Check sheet for the modelled part. Datum: model origin and axes. Units: mm. Give positions to 0.01 mm unless a question says otherwise; leave off trailing zeros. Loops run counter-clockwise (first coordinate to the right, second up) from the corner with the lowest first, then second, coordinate; pieces in that order, holes last. Notation, with made-up numbers: M 44,89.5 L 95,89.5 A6 ccw 95,95.5 Z; hole C -25.5,-27.75 d9. An arc over 180 degrees is marked long. Use one line per item in the form item = value.
from build123d import *

# Parameters (mm, degrees)
SKETCH1_R           = 67.5
SKETCH1_R_2         = 2.5
BOSS_EXTRUDE1_DEPTH = 7
SKETCH3_R           = 3
CUT_EXTRUDE1_DEPTH  = 10


with BuildPart() as part:
    # Sketch1 → Boss-Extrude1 (new body)
    with BuildSketch(Plane(origin=(0, 0, 0), x_dir=(1, 0, 0), z_dir=(0, 1, 0))):
        with Locations(Location((0, 0, 0), (0, 0, 270))):
            Circle(SKETCH1_R)
        with Locations(Location((-40, 23.094010768, 0), (0, 0, 270))):
            Circle(SKETCH1_R_2, mode=Mode.SUBTRACT)
        with Locations(Location((40, 23.094010768, 0), (0, 0, 270))):
            Circle(SKETCH1_R_2, mode=Mode.SUBTRACT)
        with Locations(Location((0, -46.188021535, 0), (0, 0, 270))):
            Circle(SKETCH1_R_2, mode=Mode.SUBTRACT)
    extrude(amount=BOSS_EXTRUDE1_DEPTH)

    # Sketch3 → Cut-Extrude1 (cut)
    with BuildSketch(Plane(origin=(0, 7, 0), x_dir=(1, 0, 0), z_dir=(0, 1, 0))):
        with Locations(Location((42.425, 42.425, 0), (0, 0, 270))):
            Circle(SKETCH3_R)
        with Locations(Location((42.425, -42.425, 0), (0, 0, 270))):
            Circle(SKETCH3_R)
        with Locations(Location((-42.425, -42.425, 0), (0, 0, 270))):
            Circle(SKETCH3_R)
        with Locations(Location((-42.425, 42.425, 0), (0, 0, 270))):
            Circle(SKETCH3_R)
    extrude(amount=-CUT_EXTRUDE1_DEPTH, mode=Mode.SUBTRACT)


solid = part.part
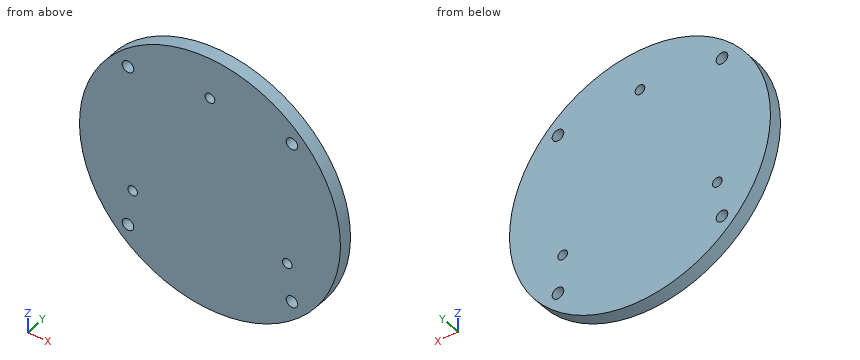
1) Section check A-A (y = 5.5). Record the cut outline in (x, z) (3 decimals), then the cut area to 3 significant figures.
Evaluation:
outline = C 0,0 d135; hole C -42.425,-42.425 d6; hole C -42.425,42.425 d6; hole C -40,-23.094 d5; hole C 0,46.188 d5; hole C 40,-23.094 d5; hole C 42.425,-42.425 d6; hole C 42.425,42.425 d6
area = 14,100 mm^2
2) Section check B-B (x = 54). Record the cut outline in (y, z), then the cut area to 3 significant figures.
Evaluation:
outline = M 0,-40.5 L 7,-40.5 L 7,40.5 L 0,40.5 Z
area = 567 mm^2
3) Depth check by flat-ended pin: pin 1 Ø4 at (x, y) = (-43, 1.5) entering from +Z; pin 2 Ø3.5 at (x, z) = (-42.425, 42.425) entering from +Y. Enter the tip coordinate at first touch or a pass-through.
Evaluation:
pin_1 = 53.62
pin_2 = through
4) Section check C-C (z = -35). Record the cut outline in (x, y).
Evaluation:
outline = M -57.72,0 L 57.72,0 L 57.72,7 L -57.72,7 Z
5) Scan lines: line 1 (X direction, y = 3, z = -43); line 2 (X direction, y = 2.5, z = -25); line 3 (X direction, y = 4.5, z = 0). Record each from-to range of solid material in increasing order.
Evaluation:
line_1 = -52.03 to -45.37, -39.48 to 39.48, 45.37 to 52.03
line_2 = -62.7 to -41.62, -38.38 to 38.38, 41.62 to 62.7
line_3 = -67.5 to 67.5
